from build123d import *

# Parameters (mm, degrees)
SKETCH1_W                    = 38.1
SKETCH1_H                    = 38.1
MAIN_BODY_DEPTH              = 34
F_9_32_RIGHT_RAIL_DEPTH      = 64.712008287
F_9_32_RIGHT_RAIL_DEPTH_BACK = 5.55625
SKETCH3_R                    = 3.571875
SKETCH4_R                    = 3.571875
F_9_32_LEFT_RAIL_DEPTH       = 5.55625
F_9_32_TOPPER_DEPTH          = 64.712008287
F_9_32_TOPPER_DEPTH_BACK     = 10
SKETCH8_R                    = 3.571875
CUT_EXTRUDE3_START           = -5.55625
CUT_EXTRUDE3_DEPTH           = 32.54375
CUT_EXTRUDE4_START           = -5.55625
CUT_EXTRUDE4_DEPTH           = 32.54375
CUT_EXTRUDE12_START          = -30.825
CUT_EXTRUDE12_OUTLINE_W      = 29.119345377
CUT_EXTRUDE12_OUTLINE_H      = 29.119345377
CUT_EXTRUDE12_DEPTH          = 22.09375
CUT_EXTRUDE15_START          = -17
CUT_EXTRUDE15_DEPTH          = 13.825
CUT_EXTRUDE16_REACH          = 65.712


# Read off the part's stored shape, not the designer's step: Cut-Extrude12
with BuildPart() as part:
    # Sketch1 → Main Body (new body)
    with BuildSketch(Plane(origin=(0, 0, 0), x_dir=(1, 0, 0), z_dir=(0, 1, 0))):
        with Locations((19.05, 19.05)):
            Rectangle(SKETCH1_W, SKETCH1_H)
    extrude(amount=MAIN_BODY_DEPTH)

    # Sketch3 → 9/32 Right Rail (cut, two sides: drawn at the far end of the back side and taken through both)
    with BuildSketch(Plane.XY.offset(-F_9_32_RIGHT_RAIL_DEPTH_BACK)):
        with Locations(Location((19.05, 17, 0), (0, 0, 180))):
            Circle(SKETCH3_R)
    extrude(amount=F_9_32_RIGHT_RAIL_DEPTH + F_9_32_RIGHT_RAIL_DEPTH_BACK, mode=Mode.SUBTRACT)

    # Sketch4 → 9/32 Left Rail (cut)
    with BuildSketch(Plane.ZY):
        with Locations((-19.05, 17)):
            Circle(SKETCH4_R)
    extrude(amount=-F_9_32_LEFT_RAIL_DEPTH, mode=Mode.SUBTRACT)

    # Sketch8 → 9/32 Topper (cut, two sides: drawn at the far end of the back side and taken through both)
    with BuildSketch(Plane(origin=(0, 34, 0), x_dir=(1, 0, 0), z_dir=(0, 1, 0)).offset(-F_9_32_TOPPER_DEPTH_BACK)):
        with Locations(Location((19.05, 19.05, 0), (0, 0, 90))):
            Circle(SKETCH8_R)
    extrude(amount=F_9_32_TOPPER_DEPTH + F_9_32_TOPPER_DEPTH_BACK, mode=Mode.SUBTRACT)

    # Sketch9 → Cut-Extrude3 (cut)
    with BuildSketch(Plane.ZY.offset(CUT_EXTRUDE3_START)):
        Polygon((-22.372470377, 22.7546875), (-25.694940754, 17), (-22.372470377, 11.2453125), (-15.727529623, 11.2453125), (-12.405059246, 17), (-15.727529623, 22.7546875), align=None)
    extrude(amount=-CUT_EXTRUDE3_DEPTH, mode=Mode.SUBTRACT)

    # Sketch10 → Cut-Extrude4 (cut)
    with BuildSketch(Plane.XY.offset(CUT_EXTRUDE4_START)):
        Polygon((15.727529623, 22.7546875), (12.405059246, 17), (15.727529623, 11.2453125), (22.372470377, 11.2453125), (25.694940754, 17), (22.372470377, 22.7546875), align=None)
    extrude(amount=-CUT_EXTRUDE4_DEPTH, mode=Mode.SUBTRACT)

    # Cut-Extrude12 outline → Cut-Extrude12 (cut)
    with BuildSketch(Plane(origin=(0, 34, 0), x_dir=(1, 0, 0), z_dir=(0, 1, 0)).offset(CUT_EXTRUDE12_START)):
        with Locations((23.540327312, 23.540327312)):
            Rectangle(CUT_EXTRUDE12_OUTLINE_W, CUT_EXTRUDE12_OUTLINE_H)
    extrude(amount=CUT_EXTRUDE12_DEPTH, mode=Mode.SUBTRACT)

    # Sketch14 → Cut-Extrude15 (cut)
    with BuildSketch(Plane(origin=(0, 34, 0), x_dir=(1, 0, 0), z_dir=(0, 1, 0)).offset(CUT_EXTRUDE15_START)):
        Polygon((23.748682668, 14.351317332), (25.468519889, 20.769837221), (20.769837221, 25.468519889), (14.351317332, 23.748682668), (12.631480111, 17.330162779), (17.330162779, 12.631480111), align=None)
    extrude(amount=CUT_EXTRUDE15_DEPTH, mode=Mode.SUBTRACT)

    # Sketch15 → Cut-Extrude16 (cut, up to next)
    with BuildSketch(Plane.XZ, mode=Mode.PRIVATE) as cut_extrude16_sk1:
        Polygon((38.1, -8.980654623), (8.980654623, -38.1), (38.1, -38.1), align=None)
    cut_extrude16_tool1 = extrude(cut_extrude16_sk1.sketch, amount=-CUT_EXTRUDE16_REACH, mode=Mode.PRIVATE) & part.part
    add(cut_extrude16_tool1.solids().sort_by_distance((28.393552, 0, -28.393552))[0], mode=Mode.SUBTRACT)


solid = part.part
Part model, mm, in its own coordinate system. A direction names the side the tool comes from. Coordinates: 2 decimals unless noted, no trailing zeros. Order: outer loops, then holes, each group sorted by start corner. A loop starts at its lowest first (then second) coordinate and runs counter-clockwise, first axis right, second up. Notation, with made-up numbers: M -5,1 L 54,1 A27 cw 54,26 Z; hole C -39.5,14.25 d4. An arc over 180 degrees is marked long. One line per question, with ' | ' between items.
Q1. 3-axis set-ups, long thin cutter, end or side, ignore diameter. For faces 1 (the face through (23, 12, -8.981)), 2 (the face through (19, 11.245, -7)), 3 (the face through (14.95, 28.01, -15.01)), 4 (the face through (5.556, 14.5, -16.2)): which of +Z, -Z, +X, -X, +Y, -Y reach the whole face in a straight line?
A:
face 1: -Z, +X | face 2: -Z | face 3: none | face 4: +X
Q2. Slice it at A-A (x = 19.05). Give the cut face in (y, z) (3 decimals), and give its area (3 significant figures).
A:
outline: M 0,-28.031 L 3.175,-28.031 L 3.175,-8.981 L 11.245,-8.981 L 11.245,-5.556 L 13.428,-5.556 L 13.428,0 L 0,0 Z; M 20.572,-5.556 L 22.755,-5.556 L 22.755,-8.981 L 25.269,-8.981 L 25.269,-13.092 L 30.825,-13.092 L 30.825,-15.478 L 34,-15.478 L 34,0 L 20.572,0 Z; M 25.269,-38.1 L 34,-38.1 L 34,-22.622 L 30.825,-22.622 L 30.825,-25.008 L 25.269,-25.008 Z | area: 452 mm^2
Q3. Drill centre lines: line 1 (Y direction, x = 14, z = -27.5) (3 decimals); line 2 (Y direction, x = 19, z = -1); line 3 (X direction, y = 17, z = -3.45). Where is each one in solid material? Low to high.
A:
line 1: y = 0 to 3.175, 25.269 to 34 | line 2: y = 0 to 13.43, 20.57 to 34 | line 3: x = 0 to 15.48, 22.62 to 38.1
Q4. Slice it at C-C (z = -19.05). Give the cut face in (x, y) (3 decimals).
A:
outline: M 0,0 L 28.031,0 L 28.031,3.175 L 8.981,3.175 L 8.981,11.245 L 5.556,11.245 L 5.556,13.428 L 0,13.428 Z; M 0,20.572 L 5.556,20.572 L 5.556,22.755 L 8.981,22.755 L 8.981,25.269 L 13.092,25.269 L 13.092,30.825 L 15.478,30.825 L 15.478,34 L 0,34 Z; M 22.622,30.825 L 25.008,30.825 L 25.008,25.269 L 38.1,25.269 L 38.1,34 L 22.622,34 Z
Q5. Slice it at B-B (y = 24). Give the cut face in (x, z), and give its area (3 significant figures).
A:
outline: M 0,-38.1 L 8.98,-38.1 L 8.98,-8.98 L 38.1,-8.98 L 38.1,0 L 0,0 Z | area: 604 mm^2
Q6. Slice it at D-D (y = 28). Give the cut face in (x, z), and give its area (3 significant figures).
A:
outline: M 0,-38.1 L 38.1,-38.1 L 38.1,0 L 0,0 Z; hole M 12.63,-17.33 L 14.35,-23.75 L 20.77,-25.47 L 25.47,-20.77 L 23.75,-14.35 L 17.33,-12.63 Z | area: 1,340 mm^2
Q7. Two-plate mould, pull along Z, no slides. Class faces 5 (the face through (23.15, 28.01, -23.09)), 6 (the face through (15, 0, -15)), 7 (the face through (19, 13, 0)), 8 (the face through (17.61, 28.01, -24.62)): +Z half, -Z half, draft (parallel to the pull), parting line (faces both ways), or undercut.
A:
face 5: undercut | face 6: draft | face 7: +Z half | face 8: undercut
Q8. Pin check, flat tips, straight feed: P1, Ø5, axis at y = 20, z = -16, coming from the +X side; P2, Ø11, axis at x = 23.5, y = 16, coming from the -Z side. Stop position of each tip, or through.
A:
P1: stops at x = 8.98 | P2: stops at z = -8.98
